```python
from build123d import *

# Parameters (mm, degrees)
SKETCH1_W           = 27.3
SKETCH1_H           = 27.3
BOSS_EXTRUDE1_DEPTH = 15
SKETCH3_W           = 35
SKETCH3_H           = 35
SKETCH3_W_2         = 27.3
SKETCH3_H_2         = 27.3
BOSS_EXTRUDE2_DEPTH = 12.6
FILLET1_R           = 1
FILLET3_R           = 3


with BuildPart() as part:
    # Sketch1 → Boss-Extrude1 (new body)
    with BuildSketch(Plane(origin=(0, 0, 0), x_dir=(1, 0, 0), z_dir=(0, 1, 0))):
        with Locations((11.5, -12.5)):
            Rectangle(SKETCH1_W, SKETCH1_H)
        Polygon((0, 0), (23, 0), (23, -14), (16.6, -25), (6.4, -25), (0, -14), align=None, mode=Mode.SUBTRACT)
    extrude(amount=BOSS_EXTRUDE1_DEPTH)

    # Sketch3 → Boss-Extrude2 (add)
    with BuildSketch(Plane(origin=(0, 0, 0), x_dir=(1, 0, 0), z_dir=(0, 1, 0))):
        with Locations((11.5, -12.5)):
            Rectangle(SKETCH3_W, SKETCH3_H)
        with Locations((11.5, -12.5)):
            Rectangle(SKETCH3_W_2, SKETCH3_H_2, mode=Mode.SUBTRACT)
    extrude(amount=BOSS_EXTRUDE2_DEPTH)

    # Fillet1
    fillet1_edges = [part.edges().sort_by_distance(p)[0] for p in [
        (0, 7.5, 0),
        (0, 7.5, 14),
        (6.4, 7.5, 25),
        (16.6, 7.5, 25),
        (23, 7.5, 14),
        (23, 7.5, 0),
    ]]
    fillet(fillet1_edges, radius=FILLET1_R)

    # Fillet3
    fillet3_edges = [part.edges().sort_by_distance(p)[0] for p in [
        (29, 6.3, 30),
        (29, 6.3, -5),
        (-6, 6.3, -5),
        (-6, 6.3, 30),
    ]]
    fillet(fillet3_edges, radius=FILLET3_R)


solid = part.part
```
Input: part model. Units: mm. Frame: model coordinates. A direction names the side the tool comes from. Give positions to 0.01 mm unless a question says otherwise; leave off trailing zeros. Loops run counter-clockwise (first coordinate to the right, second up) from the corner with the lowest first, then second, coordinate; pieces in that order, holes last.
1) Line query: L1, parallel to X at y = 12, z = 11.5; L2, parallel to Z at x = 13.5, y = 5.25; L3, parallel to Y at x = 25.5, z = 5.5. Output: solid intervals per line, ascending.
A:
L1: x = -6 to 0, 23 to 29
L2: z = -5 to 0, 25 to 30
L3: y = 0 to 12.6
2) Section query B-B on x = 11. Return the cut outline in (y, z).
A:
outline: (0, -5) - (12.6, -5) - (12.6, -1.15) - (15, -1.15) - (15, 0) - (0, 0) - close; (0, 25) - (15, 25) - (15, 26.15) - (12.6, 26.15) - (12.6, 30) - (0, 30) - close
3) Contact query for flat-ended pins moving along their axis: pin 1 (0.7 mm diameter, centred on y = 13.5, z = 11, fed in from +X); pin 2 (0.7 mm diameter, centred on y = 14, z = 6, fed in from -X). Output: stop coordinate, or through.
A:
pin 1: stops at x = 25.15
pin 2: stops at x = -2.15
4) Section query C-C on y = 4.75. Return the cut outline in (x, z), and give its area (3 significant figures).
A:
outline: (-6, -2) arc R3 ccw to (-3, -5) - (26, -5) arc R3 ccw to (29, -2) - (29, 27) arc R3 ccw to (26, 30) - (-3, 30) arc R3 ccw to (-6, 27) - close; hole (0, 1) arc R1 ccw to (1, 0) - (22, 0) arc R1 ccw to (23, 1) - (23, 13.73) arc R1 ccw to (22.86, 14.23) - (16.89, 24.5) arc R1 ccw to (16.02, 25) - (6.98, 25) arc R1 ccw to (6.11, 24.5) - (0.14, 14.23) arc R1 ccw to (0, 13.73) - close
area: 713 mm2
5) Mould query, pull axis X, two halves, no side actions, for faces 1 (the flat face through (0, 7, 7)), 2 (the flat face through (11, 7, 0)), 3 (the cylindrical face through (28.14, 6.39, -4.1)), 4 (the cylindrical face through (-5.14, 6.39, 29.1)). Classes: released by +X, released by -X, zero draft, split by the parting line, or undercut.
A:
face 1: undercut
face 2: undercut
face 3: released by +X
face 4: released by -X
6) Reachability of faces 5 (the flat face through (11, 14, -1.15)), 6 (the cylindrical face through (-5.14, 6.39, -4.1)), 7 (the flat face through (3.165, 7.395, 19.44)), 8 (the flat face through (-2.15, 14, 13)) from +Z, -Z, +X, -X, +Y, -Y: full face, straight path, thin tool, end or side. Return the list, or none.
A:
face 5: -Z, +X, -X, +Y
face 6: -Z, -X, +Y, -Y
face 7: +Y, -Y
face 8: +Z, -Z, -X, +Y
7) Section query A-A on z = 3. Return the cut outline in (x, y).
A:
outline: (-6, 0) - (0, 0) - (0, 15) - (-2.15, 15) - (-2.15, 12.6) - (-6, 12.6) - close; (23, 0) - (29, 0) - (29, 12.6) - (25.15, 12.6) - (25.15, 15) - (23, 15) - close
